Autodesk Inventor part; units mm, degrees
ref_plane "YZ Plane" through (0, 0, 0) normal (1, 0, 0) x (0, 1, 0)
ref_plane "XZ Plane" through (0, 0, 0) normal (0, 1, 0) x (-1, 0, 0)
ref_plane "XY Plane" through (0, 0, 0) normal (0, 0, 1) x (1, 0, 0)
sketch "Эскиз1" plane through (0, 0, 0) normal (0, 0, 1) x (1, 0, 0)
  circle A0 centre (0, 0) radius 7.5
  circle A1 centre (0, 0) radius 20
  circle A2 centre (0, 0) radius 22
  line L0 (0, 0) -> (-22, 0)
  line L1 (0, 0) -> (0, 22)
  line L2 (-22, 0) -> (-20, 0)
  line L3 (-20, 0) -> (-20, -4)
  line L4 (-20, -4) -> (-22, -4)
  line L5 (-22, -4) -> (-22, 0)
  point P0 (20, 0)
  point P1 (22, 0)
  point P2 (0, 20)
  point P3 (-20, 0)
  point P4 (-21.6333, -4)
  dimension "d1" = 40
  dimension "d0" = 15
  dimension "d2" = 2
  dimension "d10" = 4
extrude "Выдавливание1" add sketch "Эскиз1" along normal blind 215 contours L1 A2 L4 L3 A1 | L3 L4 A2 L0
sketch "Эскиз2" plane through (0, 0, 215) normal (0, 0, 1) x (1, 0, 0)
  arc A0 (-20, 0) -> (0, 20) centre (0, 0) ccw
  arc A1 (-22, 0) -> (0, 22) centre (0, 0) ccw
  arc A2 (-22, 0) -> (0, 22) centre (0, 0) ccw
  line L0 (0, 22) -> (0, 20)
  arc A3 (-20, 0) -> (0, 20) centre (0, 0) ccw
  line L1 (-20, 0) -> (-22, 0)
  circle A4 centre (0, 0) radius 8
  line L2 (0, 8) -> (0, 20)
  line L3 (-8, 0) -> (-20.5, 0)
  circle A5 centre (0, 0) radius 12
  point P0 (0, 20)
  point P1 (-12, 0)
  point P2 (0, 12)
  dimension "d5" = 16
  dimension "d15" = 4
extrude "Выдавливание2" add sketch "Эскиз2" against normal blind 4 contours L3 A5 L2 A0 | A5 L2 A4 L3 | L3 A4 L2 A5
sketch "Эскиз3" plane through (0, 0, 0) normal (0, 0, -1) x (-1, 0, 0)
  line L0 (20, 0) -> (12, 0)
  circle A0 centre (0, 0) radius 8
  line L1 (0, 12) -> (0, 20)
  arc A1 (0, 20) -> (20, 0) centre (0, 0) ccw
  arc A2 (12, 0) -> (0, 12) centre (0, 0) ccw
extrude "Выдавливание3" add sketch "Эскиз3" against normal blind 4
sketch "Эскиз4" plane through (0, 0, 0) normal (0, 0, -1) x (-1, 0, 0)
  arc A0 (0, 20) -> (20, 0) centre (0, 0) ccw
  line L0 (20, 0) -> (60, 0)
  line L1 (60, 0) -> (60, -4)
  line L2 (60, -4) -> (20, -4)
  line L3 (20, -4) -> (20, 0)
  dimension "d11" = 40
  dimension "d12" = 4
extrude "Выдавливание4" add sketch "Эскиз4" against normal blind 60
sketch "Эскиз5" plane through (-60, -4, 0) normal (0, -1, 0) x (1, 0, 0)
  line L0 (10, 50) -> (25, 50)
  line L1 (25, 50) -> (25, 45)
  line L2 (25, 45) -> (10, 45)
  line L3 (10, 45) -> (10, 50)
  line L4 (10, 15) -> (25, 15)
  line L5 (25, 15) -> (25, 10)
  line L6 (25, 10) -> (10, 10)
  line L7 (10, 10) -> (10, 15)
  line L8 (38.3667, 0) -> (0, 0)
  line L9 (0, 0) -> (0, 60)
  line L10 (0, 30) -> (39.4889, 30)
  line L11 (38.3667, 60) -> (38.3667, 0)
  line L12 (10, 27.5) -> (25, 27.5)
  line L13 (25, 27.5) -> (25, 32.5)
  line L14 (25, 32.5) -> (10, 32.5)
  line L15 (10, 32.5) -> (10, 27.5)
  point P0 (60, 0)
  dimension "d16" = 10
  dimension "d17" = 10
  dimension "d19" = 5
  dimension "d22" = 15
  dimension "d23" = 0
extrude "Выдавливание5" cut sketch "Эскиз5" against normal blind 10 contours L0 L1 L2 L3 | L4 L5 L6 L7 | L13 L12 L15 L10 | L10 L15 L14 L13
sketch "Эскиз6" plane through (-60, -4, 0) normal (-1, 0, 0) x (0, 0, 1)
  line L0 (211, 32.0308) -> (-1.8272, 32.0308)
  line L1 (-1.8272, 32.0308) -> (-1.8272, -28.2031)
  line L2 (-1.8272, -28.2031) -> (211, -28.2031)
  line L3 (211, -28.2031) -> (211, 32.0308)
  point P0 (0, 4)
extrude "Выдавливание6" cut sketch "Эскиз6" against normal blind 100
sketch "Эскиз7" plane through (0, 0, 211) normal (0, 0, -1) x (-1, 0, 0)
  arc A0 (0, 22) -> (22, 0) centre (0, 0) ccw
  circle A1 centre (0, 0) radius 22
  circle A2 centre (0, 0) radius 20.8
  point P0 (0, 20.8)
  point P1 (22, 0)
  dimension "d26" = 1.2
extrude "Выдавливание7" cut sketch "Эскиз7" against normal blind 2
sketch "Эскиз9" plane through (0, 0, 0) normal (0, 1, 0) x (-1, 0, 0)
  line L0 (12, 215) -> (0, 215)
  circle A0 centre (0, 215) radius 12
  line L1 (0, 215) -> (0, 227)
  line L2 (12, 215) -> (0, 227)
  point P0 (0, 0)
revolve "Вращение1" add sketch "Эскиз9" angle 360 about axis through (0, 0, 215) along (0, 0, 1) contours L0 L1 L2
sketch "Эскиз10" plane through (0, 0, 215) normal (0, 0, -1) x (-1, 0, 0)
  circle A0 centre (0, 0) radius 3
  dimension "d30" = 6
extrude "Выдавливание8" cut sketch "Эскиз10" against normal blind 5
properties part number "крышка кожуха пушки"
The listing builds one solid part. Answer for the finished solid, in the listing's coordinates (mm). A direction names the side the tool comes from. Give positions to 0.01 mm unless a question says otherwise; leave off trailing zeros. Write each loop counter-clockwise with the first axis right and the second up, starting at its lowest first coordinate (ties: lowest second). Pieces come first, ordered by that corner, then holes. Notation, with made-up numbers: (12.25, 4.5) - (31.25, 4.5) arc R18 ccw to (31.25, 24.5) - close; hole circle Ø1 at (68.25, 37.25). An arc over 180 degrees is marked (long way). Use a Markdown table: item, result.
1. Section D-D on z = 226 is taken. Write down the section's boundary in (x, y).
Values follow:
| item | result |
|---|---|
| outline | circle Ø2 at (0, 0) |
2. Section B-B on x = 15.5 is taken. Write down the section's boundary in (y, z), plus the area to 3 significant figures.
Values follow:
| item | result |
|---|---|
| outline | (-15.61, 213) - (-13.87, 213) - (-13.87, 211) - (13.87, 211) - (13.87, 213) - (15.61, 213) - (15.61, 215) - (-15.61, 215) - close |
| area | 118 mm² |
3. For a pull along X with two mould halves and no side action, classify faces 4 (the cylindrical face through (-8.39, 8.58, 213.03)), 5 (the flat face through (9, -9, 215)), 6 (the flat face through (-3.4, -0.1, 215)) as released by +X, released by -X, zero draft, split by the parting line, or undercut.
Values follow:
| item | result |
|---|---|
| face 4 | released by -X |
| face 5 | zero draft |
| face 6 | undercut |
4. A tool of negligible diameter and unlimited length cuts with its end or side. For faces 1 (the conical face through (0.74, -3.34, 223.58)), 2 (the flat face through (0, 17, 213)), 3 (the flat face through (12, -18, 213)), from which of +Z, -Z, +X, -X, +Y, -Y can it reach the whole face along a straight path? Write none if from no direction.
Values follow:
| item | result |
|---|---|
| face 1 | +Z |
| face 2 | +Z, -Z, -X, +Y |
| face 3 | -Z |
5. Find the intervals of material crossed by probe 1 along Z at (x, y) = (16.5, -10); probe 2 along Y at (x, z) = (4, 222); probe 3 along Z at (x, y) = (8, 20), in increasing order. Write a range as from..to.
Values follow:
| item | result |
|---|---|
| probe 1 | z = 211..215 |
| probe 2 | y = -3..3 |
| probe 3 | z = 213..215 |
6. Section A-A on z = 215.75 is taken. Write down the section's boundary in (x, y), plus the area to 3 significant figures.
Values follow:
| item | result |
|---|---|
| outline | circle Ø22.5 at (0, 0); hole circle Ø6 at (0, 0) |
| area | 369 mm² |
7. Each of these flat-tipped pins is pushed along its axis until it touches: P1, Ø8, axis at x = 3, z = 223.5, coming from the -Y side; P2, Ø3, axis at x = -6.5, z = 219, coming from the -Y side; P3, Ø3, axis at y = 18.5, z = 212.5, coming from the -X side. Where does it stop, or does it pass through?
Values follow:
| item | result |
|---|---|
| P1 | stops at y = -7.1 |
| P2 | stops at y = -7.31 |
| P3 | stops at x = 0 |
